Work out the finished part from the listing and answer in its coordinate system (mm). Coordinates: 2 decimals unless noted, no trailing zeros. Order: outer loops, then holes, each group sorted by start corner. A loop starts at its lowest first (then second) coordinate and runs counter-clockwise, first axis right, second up.
1. Find the intervals of material crossed by probe 1 along Y at (x, z) = (0.25, 4.5); probe 2 along X at (y, z) = (12.75, 2.25); probe 3 along Y at (x, z) = (-7.5, -2), in increasing order.
2. The part is cut by section D-D, the plane z = 0. Give the vertices of the cut face in (x, y), then the cut area to 3 significant figures.
3. Determine the mould class of faces 1 (the cylindrical face through (0.15, 24.4, 11.93)), 2 (the cylindrical face through (10, 15.7, 0.2)), 3 (the flat face through (-5, 3, -12.5)) for opening direction Y: +Y half, -Y half, draft (parallel to the pull), parting line (faces both ways), or undercut.
4. The part is cut by section A-A, the plane x = 0. Count the separate pieces of the cut face and the enclosed holes in it, then the cut area to 3 significant figures.
5. The part is cut by section B-B, the plane z = -8. Give the vertices of the cut face in (x, y), then the cut area to 3 significant figures.
```python
from build123d import *

# Parameters (mm, degrees)
SKETCH1_W           = 25
SKETCH1_H           = 25
BOSS_EXTRUDE1_DEPTH = 25
SKETCH2_R           = 10.5
CUT_EXTRUDE1_DEPTH  = 25
CUT_EXTRUDE2_REACH  = 32.619
SKETCH3_R           = 2.5
FILLET1_R           = 2


with BuildPart() as part:
    # Sketch1 → Boss-Extrude1 (new body)
    with BuildSketch(Plane(origin=(0, 0, 0), x_dir=(1, 0, 0), z_dir=(0, 1, 0))):
        Rectangle(SKETCH1_W, SKETCH1_H)
    extrude(amount=BOSS_EXTRUDE1_DEPTH)

    # Sketch2 → Cut-Extrude1 (cut)
    with BuildSketch(Plane.XY.offset(12.5)):
        with Locations((0, 12.5)):
            Circle(SKETCH2_R)
    extrude(amount=-CUT_EXTRUDE1_DEPTH, mode=Mode.SUBTRACT)

    # Cut-Extrude2: up to this face of the body (flat: up to its plane)
    cut_extrude2_end = Plane(part.part.faces().sort_by_distance((0, 0, 0))[0])
    # Sketch3 → Cut-Extrude2 (cut, up to the picked face)
    with BuildSketch(Plane(origin=(0, 25, 0), x_dir=(1, 0, 0), z_dir=(0, 1, 0)), mode=Mode.PRIVATE) as cut_extrude2_sk1:
        with Locations(Location((0, 0, 0), (0, 0, 270))):
            Circle(SKETCH3_R)
    cut_extrude2_tool1 = split(extrude(cut_extrude2_sk1.sketch, amount=-CUT_EXTRUDE2_REACH, mode=Mode.PRIVATE), bisect_by=cut_extrude2_end, keep=Keep.BOTH, mode=Mode.PRIVATE)
    add(cut_extrude2_tool1.solids().sort_by(Axis((0, 25, 0), (0, -1, 0)))[0], mode=Mode.SUBTRACT)

    # Fillet1
    fillet1_edges = [part.edges().sort_by_distance(p)[0] for p in [
        (12.5, 25, 0),
        (0, 25, -12.5),
        (-12.5, 25, 0),
        (0, 0, -12.5),
        (12.5, 0, 0),
        (0, 0, 12.5),
        (-12.5, 0, 0),
        (-12.5, 12.5, -12.5),
        (12.5, 12.5, -12.5),
        (12.5, 12.5, 12.5),
        (-12.5, 12.5, 12.5),
        (0, 25, 12.5),
    ]]
    fillet(fillet1_edges, radius=FILLET1_R - 0.0001)  # a hair under: the kernel refuses the full size


solid = part.part
```
Geometry says:
1. probe 1: y = 0 to 2, 23 to 25
1. probe 2: x = -12.5 to -10.5, 10.5 to 12.5
1. probe 3: y = 0 to 5.15, 19.85 to 25
2. outline: (-12.5, 2) arc R2 ccw to (-10.5, 0) - (-2.5, 0) - (-2.5, 2.3) arc R10.5 cw to (-2.5, 22.7) - (-2.5, 25) - (-10.5, 25) arc R2 ccw to (-12.5, 23) - close; (2.5, 0) - (10.5, 0) arc R2 ccw to (12.5, 2) - (12.5, 23) arc R2 ccw to (10.5, 25) - (2.5, 25) - (2.5, 22.7) arc R10.5 cw to (2.5, 2.3) - close
2. area: 254 mm2
3. face 1: +Y half
3. face 2: undercut
3. face 3: draft
4. separate pieces: 4
4. enclosed holes: 0
4. area: 76.6 mm2
5. outline: (-12.5, 2) arc R2 ccw to (-10.5, 0) - (10.5, 0) arc R2 ccw to (12.5, 2) - (12.5, 23) arc R2 ccw to (10.5, 25) - (-10.5, 25) arc R2 ccw to (-12.5, 23) - close; hole circle Ø21 at (0, 12.5)
5. area: 275 mm2
